Source: three-view drawing plus pictorial views. Frame: mm from the lowest corner of the part. A direction names the side the tool comes from. Give positions to 0.01 mm unless a question says otherwise; leave off trailing zeros. Write each loop counter-clockwise with the first axis right and the second up, starting at its lowest first coordinate (ties: lowest second). Pieces come first, ordered by that corner, then holes. Notation, with made-up numbers: M 15,-0.75 L 54,-0.75 A28 ccw 54,23.25 Z; hole C 41.25,36 d2. An arc over 180 degrees is marked long. One line per question, with ' | ' between items.
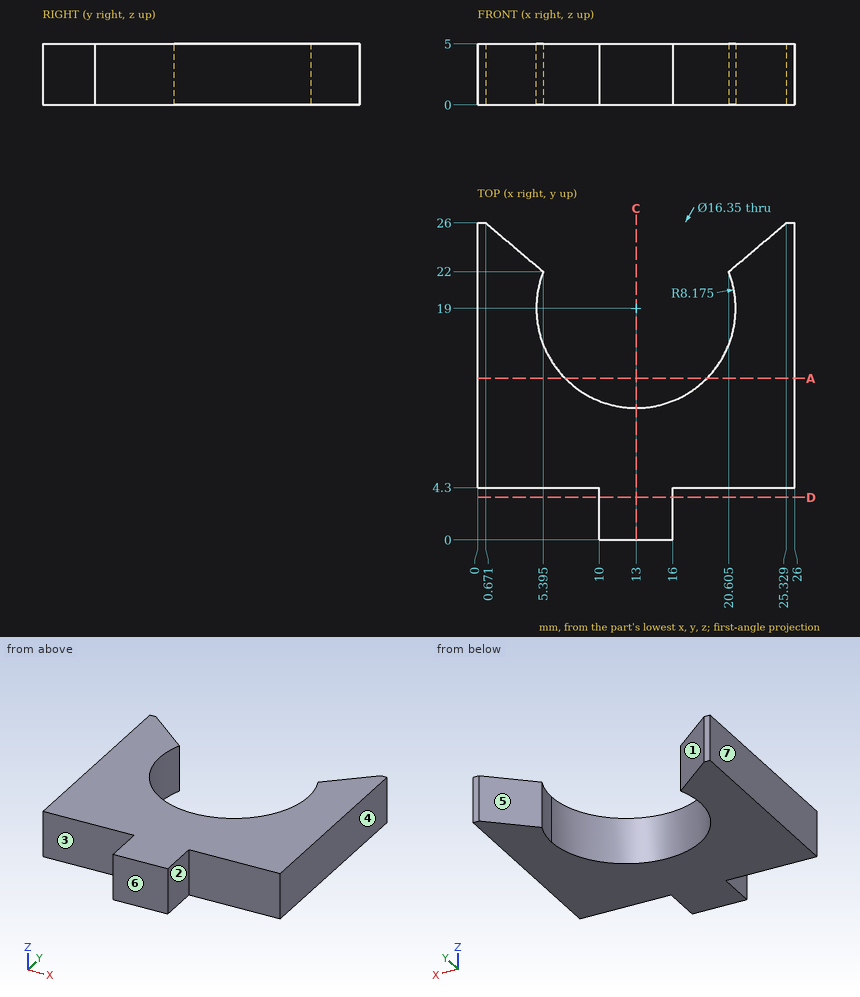
(1) Set-up query: the marked faces 1, 2, 3 and 4. Return all of +Z, -Z, +X, -X, +Y, -Y with unobstructed straight access to the full face (end or side cutting, diameter ignored); none if empty.
Working result:
face 1: +Z, -Z, +Y | face 2: +Z, -Z, +X, -Y | face 3: +Z, -Z, -X, -Y | face 4: +Z, -Z, +X, +Y, -Y
(2) Cut plane A-A, the plane y = 13.25. Return loops of the section in (x, z), then the cut area to 3 significant figures.
Working result:
outline: M 0,0 L 7.19,0 L 7.19,5 L 0,5 Z; M 18.81,0 L 26,0 L 26,5 L 18.81,5 Z | area: 71.9 mm^2
(3) First-contact query: P1, Ø1.3, axis at y = 2, z = 1.5, coming from the +X side; P2, Ø2, axis at y = 1.5, z = 3.5, coming from the -X side; P3, Ø2, axis at x = 13, z = 4, coming from the +Y side. Flat tips, straight axial feed; report the tip coordinate or a pass-through.
Working result:
P1: stops at x = 16 | P2: stops at x = 10 | P3: stops at y = 10.89
(4) Cut plane C-C, the plane x = 13. Return loops of the section in (y, z) (1 decimal).
Working result:
outline: M 0,0 L 10.8,0 L 10.8,5 L 0,5 Z
(5) Cut plane D-D, the plane y = 3.5. Return loops of the section in (x, z).
Working result:
outline: M 10,0 L 16,0 L 16,5 L 10,5 Z
(6) Material intervals for L1, parallel to X at y = 19, z = 1.3 (1 decimal); L2, parallel to Y at x = 13, z = 3.1 (1 decimal); L3, parallel to X at y = 1.5, z = 0.7, sorted ascending. Write a range as [from, to].
Working result:
L1: x = [0, 4.8], [21.2, 26] | L2: y = [0, 10.8] | L3: x = [10, 16]
(7) Draft query along X for the marked faces 5, 6 and 7. Return one class per face: released by +X, released by -X, zero draft, split by the parting line, or undercut.
Working result:
face 5: undercut | face 6: zero draft | face 7: released by -X
